Work out the finished part from the listing and answer in its coordinate system (mm). A direction names the side the tool comes from. Give positions to 0.01 mm unless a question says otherwise; leave off trailing zeros. Loops run counter-clockwise (first coordinate to the right, second up) from the corner with the lowest first, then second, coordinate; pieces in that order, holes last. Notation, with made-up numbers: (-9.75, 9) -> (48.25, 9) arc R20 ccw to (48.25, 29) -> close; hole circle Ø10 at (53.5, 0.5). An arc over 180 degrees is marked (long way). Answer as CSV lines item,"result". Start each with the question number.
1. Find section B-B, the plane x = 0. Give the vertices of the cut face in (y, z), and give its area (4 significant figures).
2. Find the intervals of material crossed by line 1 along Y through (x, z) = (0, 6.5); line 2 along X through (y, z) = (0, 6.45); line 3 along Y through (x, z) = (0, 3.1), in increasing order.
3. Determine the mould class of faces 4 (the face through (6.772, 17.035, 5.028)), 5 (the face through (0, -5, 7)), 6 (the face through (13, -25, 3)), 7 (the face through (13, 25, 5)) for opening direction Y: +Y half, -Y half, draft (parallel to the pull), parting line (faces both ways), or undercut.
4. Flat-ended cylindrical pins translate along their axes: pin 1 Ø12.5 at (x, y) = (-0.5, 13.5) entering from -Z; pin 2 Ø2.5 at (x, z) = (-12.5, 1) entering from +Y; pin 3 Ø7 at (x, y) = (3, 5.5) entering from -Z; pin 4 Ø7 at (x, y) = (0, 0) entering from +Z. Find the tip coordinate at first contact, or state that the pin passes through.
5. Find section C-C, the plane y = 15.3. Give the vertices of the cut face in (x, z).
6. Find section A-A, the plane z = 4.5. Give the vertices of the cut face in (x, y).
7. A tool of negligible diameter and unlimited length cuts with its end or side. For faces 1 (the face through (-5, 0, 5)), 2 (the face through (0, -15, 0)), 3 (the face through (0, 15, 3)), from which of +Z, -Z, +X, -X, +Y, -Y can it reach the whole face along a straight path? Write none if from no direction.
8. Find section D-D, the plane z = 2. Give the vertices of the cut face in (x, y), and give its area (3 significant figures).
from build123d import *

# Parameters (mm, degrees)
SKETCH_1_R          = 4
EXTRUDE_1_DEPTH     = 7
SKETCH_3_R          = 1.75
CUT_EXTRUDE_2_DEPTH = 10
CUT_EXTRUDE_4_DEPTH = 3
SKETCH_6_R          = 11.25
CUT_EXTRUDE_5_DEPTH = 5


with BuildPart() as part:
    # Эскиз1 → Бобышка-Вытянуть1 (new body)
    with BuildSketch(Plane.XY):
        with BuildLine():
            Line((-15, -25), (-10.077822185, -25))
            ThreePointArc((-10.077822185, -25), (0, -18.75), (10.077822185, -25))
            Line((10.077822185, -25), (15, -25))
            Line((15, -25), (15, 25))
            Line((15, 25), (10.077822185, 25))
            ThreePointArc((10.077822185, 25), (0, 18.75), (-10.077822185, 25))
            Line((-10.077822185, 25), (-15, 25))
            Line((-15, 25), (-15, -25))
        make_face()
        Circle(SKETCH_1_R, mode=Mode.SUBTRACT)
    extrude(amount=EXTRUDE_1_DEPTH)

    # Эскиз3 → Вырез-Вытянуть2 (cut)
    with BuildSketch(Plane.XY.offset(7)):
        with Locations((-10, 15.3)):
            Circle(SKETCH_3_R)
        with Locations((7, 15.3)):
            Circle(SKETCH_3_R)
    extrude(amount=-CUT_EXTRUDE_2_DEPTH, mode=Mode.SUBTRACT)

    # Эскиз4 → Вырез-Вытянуть4 (cut)
    with BuildSketch(Plane(origin=(0, 0, 0), x_dir=(-1, 0, 0), z_dir=(0, 0, -1))):
        with BuildLine():
            Line((-15, 0), (-4, 0))
            ThreePointArc((-4, 0), (0, 4), (4, 0))
            Line((4, 0), (15, 0))
            Line((15, 0), (15, 25))
            Line((15, 25), (-15, 25))
            Line((-15, 25), (-15, 0))
        make_face()
    extrude(amount=-CUT_EXTRUDE_4_DEPTH, mode=Mode.SUBTRACT)

    # Эскиз6 → Вырез-Вытянуть5 (cut)
    with BuildSketch(Plane(origin=(0, 0, 0), x_dir=(-1, 0, 0), z_dir=(0, 0, -1))):
        Circle(SKETCH_6_R)
    extrude(amount=-CUT_EXTRUDE_5_DEPTH, mode=Mode.SUBTRACT)


solid = part.part
Resolved:
1,outline,"(-18.75, 0) -> (-11.25, 0) -> (-11.25, 5) -> (-4, 5) -> (-4, 7) -> (-18.75, 7) -> close; (4, 5) -> (11.25, 5) -> (11.25, 3) -> (18.75, 3) -> (18.75, 7) -> (4, 7) -> close"
1,area,"111.5 mm^2"
2,line 1,"y = -18.75 to -4, 4 to 18.75"
2,line 2,"x = -15 to -4, 4 to 15"
2,line 3,"y = -18.75 to -11.25, 11.25 to 18.75"
3,face 4,"undercut"
3,face 5,"draft"
3,face 6,"-Y half"
3,face 7,"+Y half"
4,pin 1,"stops at z = 3"
4,pin 2,"stops at y = 0"
4,pin 3,"stops at z = 5"
4,pin 4,"passes through"
5,outline,"(-15, 3) -> (-11.75, 3) -> (-11.75, 7) -> (-15, 7) -> close; (-8.25, 3) -> (5.25, 3) -> (5.25, 7) -> (-8.25, 7) -> close; (8.75, 3) -> (15, 3) -> (15, 7) -> (8.75, 7) -> close"
6,outline,"(-15, -25) -> (-10.08, -25) arc R11.25 cw to (10.08, -25) -> (15, -25) -> (15, 25) -> (10.08, 25) arc R11.25 cw to (-10.08, 25) -> (-15, 25) -> close; hole circle Ø3.5 at (-10, 15.3); hole circle Ø22.5 at (0, 0); hole circle Ø3.5 at (7, 15.3)"
7,face 1,"-Z"
7,face 2,"-Z, +X, -X, +Y, -Y"
7,face 3,"-Z, +X, -X, +Y"
8,outline,"(-15, -25) -> (-10.08, -25) arc R11.25 cw to (10.08, -25) -> (15, -25) -> (15, 0) -> (11.25, 0) arc R11.25 cw to (-11.25, 0) -> (-15, 0) -> close"
8,area,"461 mm^2"
